```python
from build123d import *

# Parameters (mm, degrees)
SKETCH_1_R      = 6
EXTRUDE_1_DEPTH = 25
EXTRUDE_2_DEPTH = 5
FILLET_1_R      = 1
FILLET_2_R      = 0.5


with BuildPart() as part:
    # 草图1 → 凸台-拉伸1 (new body)
    with BuildSketch(Plane.XY):
        Circle(SKETCH_1_R)
    extrude(amount=EXTRUDE_1_DEPTH)

    # 草图3 → 凸台-拉伸2 (add)
    with BuildSketch(Plane.XY.offset(25)):
        Polygon((5.773502692, -10), (11.547005384, 0), (5.773502692, 10), (-5.773502692, 10), (-11.547005384, 0), (-5.773502692, -10), align=None)
    extrude(amount=-EXTRUDE_2_DEPTH)

    # 圆角1
    fillet_1_edges = [part.edges().sort_by_distance(p)[0] for p in [
        (0, -10, 25),
        (8.660254038, -5, 25),
        (8.660254038, 5, 25),
        (0, 10, 25),
        (-8.660254038, 5, 25),
        (-8.660254038, -5, 25),
    ]]
    fillet(fillet_1_edges, radius=FILLET_1_R)

    # 圆角2
    fillet_2_edges = [part.edges().sort_by_distance(p)[0] for p in [
        (-6, 0, 0),
    ]]
    fillet(fillet_2_edges, radius=FILLET_2_R)


solid = part.part
```
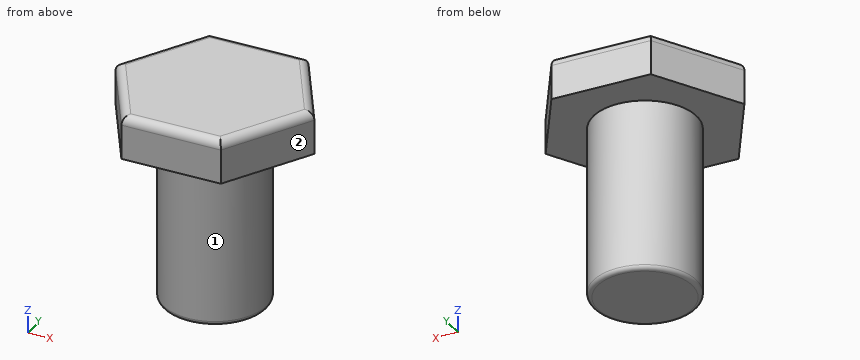
For this review, take the finished solid that the model builds, in its own axes (mm). Face numbers are marked on the shaded views. A direction names the side the tool comes from. Coordinates: 2 decimals unless noted, no trailing zeros. Loops run counter-clockwise (first coordinate to the right, second up) from the corner with the lowest first, then second, coordinate; pieces in that order, holes last. Notation, with made-up numbers: (77.5, -33.5) -> (82.5, -33.5) arc R22 ccw to (82.5, -15.5) -> close; hole circle Ø6 at (83, 56.5). An arc over 180 degrees is marked (long way). Return JSON: item names as keys, results as strings. Group by question number.
(1) Consider section A-A, the plane x = 0. Give the boundary of the cut face in (y, z), plus the area to 3 significant figures.
(2) Tool access review of the marked faces 1 and 2: name each direction out of +Z, -Z, +X, -X, +Y, -Y from which nothing blocks a thin tool from reaching the whole face with its end or side.
(3) For pin 1 Ø1 at (x, y) = (-1, 6.5) entering from -Z; pin 2 Ø6 at (y, z) = (-1.5, 6.5) entering from +X; pin 3 Ø1.5 at (x, z) = (-5, 8) entering from -Y, all flat-tipped, find the tip position at first contact; note any pin that passes through.
(4) Consider section B-B, the plane z = 5. Give the boundary of the cut face in (x, y).
(5) To check wall thickness, follow L1, parallel to Z at x = 6, y = 2.75; L2, parallel to Y at x = 0.25, z = 9.5; L3, parallel to X at y = -0.5, z = 15.75. State the ranges of each line that lie inside material, in increasing order.
Results below:
{
 "1": {"outline": "(-10, 20) -> (-6, 20) -> (-6, 0.5) arc R0.5 ccw to (-5.5, 0) -> (5.5, 0) arc R0.5 ccw to (6, 0.5) -> (6, 20) -> (10, 20) -> (10, 24) arc R1 ccw to (9, 25) -> (-9, 25) arc R1 ccw to (-10, 24) -> close", "area": "339 mm2"},
 "2": {"face 1": "-Z", "face 2": "+Z, -Z, +X, -Y"},
 "3": {"pin 1": "stops at z = 20", "pin 2": "stops at x = 6", "pin 3": "stops at y = -4.24"},
 "4": {"outline": "circle Ø12 at (0, 0)"},
 "5": {"L1": "z = 20 to 25", "L2": "y = -5.99 to 5.99", "L3": "x = -5.98 to 5.98"}
}
